Source: CAD feature listing. Evaluate the final solid. Frame: model axes, mm. Face numbers are marked on the shaded views. A direction names the side the tool comes from. Give positions to 0.01 mm unless a question says otherwise; leave off trailing zeros. Write each loop counter-clockwise with the first axis right and the second up, starting at its lowest first coordinate (ties: lowest second). Pieces come first, ordered by that corner, then holes. Notation, with made-up numbers: M 65.5,-21.5 L 83.5,-21.5 A17 cw 83.5,6.5 Z; hole C 13.5,-38 d6. An arc over 180 degrees is marked long. Return JSON: item names as keys, results as strings.
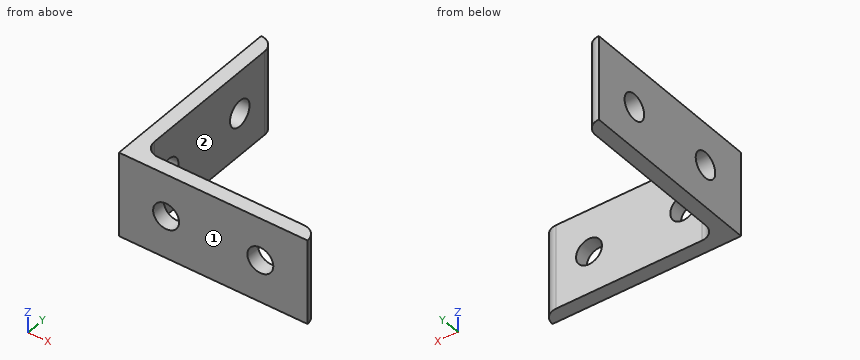
```python
from build123d import *

# Parameters (mm, degrees)
BOSS_EXTRUDE1_DEPTH = 9
SKETCH2_R           = 2.75
CUT_EXTRUDE1_DEPTH  = 41
SKETCH3_R           = 2.75
CUT_EXTRUDE2_DEPTH  = 41


with BuildPart() as part:
    # Sketch1 → Boss-Extrude1 (new body, symmetric)
    with BuildSketch(Plane.XY):
        with BuildLine():
            Line((0, 0), (0, 40))
            ThreePointArc((0, 40), (2.121320344, 39.121320344), (3, 37))
            Line((3, 37), (3, 6))
            ThreePointArc((3, 6), (3.878679656, 3.878679656), (6, 3))
            Line((6, 3), (37, 3))
            ThreePointArc((37, 3), (39.121320344, 2.121320344), (40, 0))
            Line((40, 0), (0, 0))
        make_face()
    extrude(amount=BOSS_EXTRUDE1_DEPTH, both=True)

    # Sketch2 → Cut-Extrude1 (cut, through all)
    with BuildSketch(Plane(origin=(0, 0, 0), x_dir=(1, 0, 0), z_dir=(0, 1, 0))):
        with Locations((10, 0)):
            Circle(SKETCH2_R)
        with Locations((30, 0)):
            Circle(SKETCH2_R)
    extrude(amount=CUT_EXTRUDE1_DEPTH, mode=Mode.SUBTRACT)

    # Sketch3 → Cut-Extrude2 (cut, through all)
    with BuildSketch(Plane(origin=(0, 0, 0), x_dir=(0, 0, -1), z_dir=(1, 0, 0))):
        with Locations((0, 10)):
            Circle(SKETCH3_R)
        with Locations((0, 30)):
            Circle(SKETCH3_R)
    extrude(amount=CUT_EXTRUDE2_DEPTH, mode=Mode.SUBTRACT)


solid = part.part
```
1) Set-up query: the marked faces 1 and 2. Return all of +Z, -Z, +X, -X, +Y, -Y with unobstructed straight access to the full face (end or side cutting, diameter ignored); none if empty.
Numbers:
{"face 1": "+Z, -Z, +X, -X, -Y", "face 2": "+Z, -Z, +X, +Y"}
2) Cut plane A-A, the plane y = 30. Return the cut outline in (x, z).
Numbers:
{"outline": "M 0,-9 L 3,-9 L 3,-2.75 L 0,-2.75 Z; M 0,2.75 L 3,2.75 L 3,9 L 0,9 Z"}
3) Line query: line 1 (Y direction, x = 1.2, z = 0); line 2 (Z direction, x = 30, y = 1.95); line 3 (X direction, y = 1.65, z = 0). Output: solid intervals per line, ascending. Write a range as [from, to].
Numbers:
{"line 1": "y = [0, 7.25], [12.75, 27.25], [32.75, 39.75]", "line 2": "z = [-9, -2.75], [2.75, 9]", "line 3": "x = [0, 7.25], [12.75, 27.25], [32.75, 39.51]"}
4) Contact query for flat-ended pins moving along their axis: pin 1 Ø1 at (y, z) = (10.5, -2.5) entering from +X; pin 2 Ø7 at (x, z) = (30, 0) entering from +Y; pin 3 Ø3.5 at (y, z) = (10, 0) entering from -X (3 decimals). Output: stop coordinate, or through.
Numbers:
{"pin 1": "stops at x = 3", "pin 2": "stops at y = 3", "pin 3": "passes through"}
5) Cut plane C-C, the plane z = 2.25. Return the cut outline in (x, y), then the cut area to 3 significant figures.
Numbers:
{"outline": "M 0,0 L 8.42,0 L 8.42,3 L 6,3 A3 cw 3,6 L 3,8.42 L 0,8.42 Z; M 0,11.58 L 3,11.58 L 3,28.42 L 0,28.42 Z; M 0,31.58 L 3,31.58 L 3,37 A3 ccw 0,40 Z; M 11.58,0 L 28.42,0 L 28.42,3 L 11.58,3 Z; M 31.58,0 L 40,0 A3 ccw 37,3 L 31.58,3 Z", "area": "191 mm²"}
6) Cut plane D-D, the plane z = 8. Return the cut outline in (x, y), then the cut area to 3 significant figures.
Numbers:
{"outline": "M 0,0 L 40,0 A3 ccw 37,3 L 6,3 A3 cw 3,6 L 3,37 A3 ccw 0,40 Z", "area": "229 mm²"}
